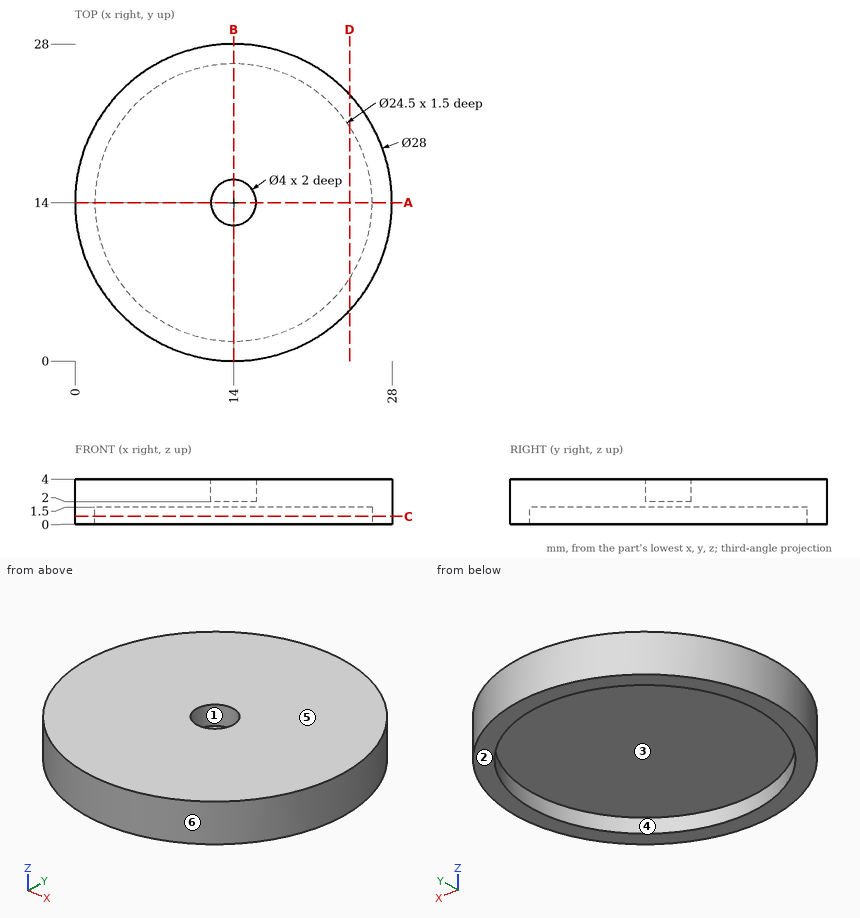
Print and shaded views of the part. All mm, measured from the part's lowest x, y and z. A direction names the side the tool comes from. Give positions to 0.01 mm unless a question says otherwise; leave off trailing zeros. Order: outer loops, then holes, each group sorted by start corner. A loop starts at its lowest first (then second) coordinate and runs counter-clockwise, first axis right, second up. Notation, with made-up numbers: (-39.75, 76) - (7.25, 76) arc R11 cw to (7.25, 86) - close; hole circle Ø6 at (73, -18.75). An arc over 180 degrees is marked (long way). Use a Markdown table: item, result.
1) Two-plate mould, pull along Y, no slides. Class the marked faces 4, 5 and 6: +Y half, -Y half, draft (parallel to the pull), parting line (faces both ways), or undercut.
Checked values:
| item | result |
|---|---|
| face 4 | undercut |
| face 5 | draft |
| face 6 | parting line |
2) Flat gauge pins, fed straight in: P1, Ø1, axis at x = 19.5, z = 3.5, coming from the +Y side; P2, Ø1.5, axis at x = 9.5, y = 7.5, coming from the -Z side; P3, Ø2, axis at x = 13.5, y = 14.5, coming from the +Z side. Where does each tip first touch, or does it go through?
Checked values:
| item | result |
|---|---|
| P1 | y = 27.08 |
| P2 | z = 1.5 |
| P3 | z = 2 |
3) Saw through at D-D on x = 24.25. List the corners of the cut face in (y, z), plus the area to 3 significant figures.
Checked values:
| item | result |
|---|---|
| outline | (4.46, 0) - (7.29, 0) - (7.29, 1.5) - (20.71, 1.5) - (20.71, 0) - (23.54, 0) - (23.54, 4) - (4.46, 4) - close |
| area | 56.2 mm² |
4) Saw through at A-A on y = 14. List the corners of the cut face in (x, z).
Checked values:
| item | result |
|---|---|
| outline | (0, 0) - (1.75, 0) - (1.75, 1.5) - (26.25, 1.5) - (26.25, 0) - (28, 0) - (28, 4) - (16, 4) - (16, 2) - (12, 2) - (12, 4) - (0, 4) - close |
5) Saw through at C-C on z = 0.7. List the corners of the cut face in (x, y).
Checked values:
| item | result |
|---|---|
| outline | circle Ø28 at (14, 14); hole circle Ø24.5 at (14, 14) |
6) Probe L1, parallel to Y at x = 14, z = 0.95; L2, parallel to Y at x = 14, z = 3; L3, parallel to Z at x = 13.5, y = 8. List the from-to ranges inside material, lowest first. Write a range as from..to.
Checked values:
| item | result |
|---|---|
| L1 | 0..1.75, 26.25..28 |
| L2 | 0..12, 16..28 |
| L3 | 1.5..4 |
7) 3-axis set-ups, long thin cutter, end or side, ignore diameter. For the marked faces 1, 2 and 3: which of +Z, -Z, +X, -X, +Y, -Y reach the whole face in a straight line?
Checked values:
| item | result |
|---|---|
| face 1 | +Z |
| face 2 | -Z, +X, -X, +Y, -Y |
| face 3 | -Z |
